CAD build for the part. Positions are in the model's coordinates, mm. Face numbers are marked on the shaded views. Round coordinates to 2 decimals unless told otherwise and drop trailing zeros. Loops run counter-clockwise (first coordinate to the right, second up) from the corner with the lowest first, then second, coordinate; pieces in that order, holes last. Notation, with made-up numbers: M 42.5,38 L 86.5,38 A37 ccw 86.5,75 Z; hole C -31.5,39.5 d8. An arc over 180 degrees is marked long. Use a Markdown table: item, result. Add a question column.
(1) Wall check: L1, parallel to Y at x = 33.25, z = 2.2; L2, parallel to Y at x = 23.5, z = 2.15; L3, parallel to X at y = -0.5, z = 2.8. Give the ranges that are in metal, low to high.
(2) Two-plate mould, pull along Y, no slides. Class the marked faces 1 and 2: released by +Y, released by -Y, zero draft, split by the parting line, or undercut.
(3) Band-saw the part on B-B, the plane x = 33.05. Write the cut outline in (y, z), and give its area (3 significant figures).
(4) Band-saw the part on D-D, the plane x = 12. Write the cut outline in (y, z), and give its area (3 significant figures).
(5) Band-saw the part on C-C, the plane z = 2.3. Give the number of separate pieces and of enclosed holes in the cut face, and give its area (3 significant figures).
(6) Band-saw the part on A-A, the plane y = -6. Write the cut outline in (x, z), and give its area (3 significant figures).
(7) Flat gauge pins, fed straight in: P1, Ø1.5, axis at y = -6, z = 1.5, coming from the -X side; P2, Ø1.5, axis at x = 39.5, z = 1.5, coming from the -Y side; P3, Ø1.5, axis at y = -5, z = 2, coming from the +X side. Where does each tip first touch, or does it go through?
from build123d import *

# Parameters (mm, degrees)
ESBO_O1_R                = 1.5
ESBO_O1_W                = 11
ESBO_O1_H                = 5.2
RESSALTO_EXTRUS_O1_DEPTH = 3
FILETE1_R                = 1.5
FILETE2_R                = 1.5


with BuildPart() as part:
    # Esboço1 → Ressalto-extrusão1 (new body)
    with BuildSketch(Plane.XY):
        with BuildLine():
            Line((0, 10.916708968), (0, 0))
            Line((0, 0), (3.1, 0))
            Line((3.1, 0), (3.1, -9))
            Line((3.1, -9), (11.2, -9))
            Line((11.2, -9), (11.2, 0))
            Line((11.2, 0), (29.2, 0))
            Line((29.2, 0), (29.2, -9))
            Line((29.2, -9), (37.3, -9))
            Line((37.3, -9), (37.3, 0))
            Line((37.3, 0), (40.4, 0))
            Line((40.4, 0), (40.4, 10.916708968))
            ThreePointArc((40.4, 10.916708968), (25, 14.2), (40.4, 17.483291032))
            Line((40.4, 17.483291032), (40.4, 28.4))
            Line((40.4, 28.4), (0, 28.4))
            Line((0, 28.4), (0, 17.483291032))
            ThreePointArc((0, 17.483291032), (9.028541033, 22.073055315), (15.4, 14.2))
            ThreePointArc((15.4, 14.2), (9.028541033, 6.326944685), (0, 10.916708968))
        make_face()
        with Locations((7.15, -6)):
            Circle(ESBO_O1_R, mode=Mode.SUBTRACT)
        with Locations((20.2, 6.6)):
            Rectangle(ESBO_O1_W, ESBO_O1_H, mode=Mode.SUBTRACT)
        with Locations((33.25, -6)):
            Circle(ESBO_O1_R, mode=Mode.SUBTRACT)
        with Locations((20.2, 21.8)):
            Rectangle(ESBO_O1_W, ESBO_O1_H, mode=Mode.SUBTRACT)
    extrude(amount=RESSALTO_EXTRUS_O1_DEPTH)

    # Filete1
    filete1_edges = [part.edges().sort_by_distance(p)[0] for p in [
        (14.7, 24.4, 1.5),
        (14.7, 19.2, 1.5),
        (25.7, 19.2, 1.5),
        (25.7, 24.4, 1.5),
    ]]
    fillet(filete1_edges, radius=FILETE1_R)

    # Filete2
    filete2_edges = [part.edges().sort_by_distance(p)[0] for p in [
        (25.7, 9.2, 1.5),
        (14.7, 9.2, 1.5),
        (14.7, 4, 1.5),
        (25.7, 4, 1.5),
    ]]
    fillet(filete2_edges, radius=FILETE2_R)


solid = part.part
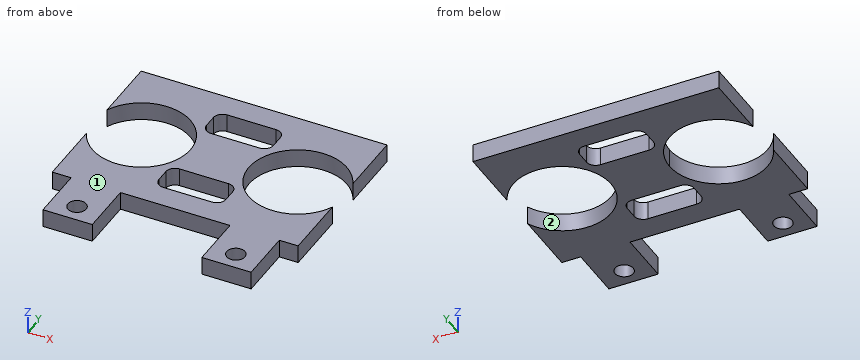
Return value:
| question | item | result |
|---|---|---|
| 1 | L1 | -9 to -7.5, -4.5 to 6.15, 22.25 to 28.4 |
| 1 | L2 | 0 to 4, 9.2 to 19.2, 24.4 to 28.4 |
| 1 | L3 | 3.1 to 11.2, 29.2 to 37.3 |
| 2 | face 1 | zero draft |
| 2 | face 2 | undercut |
| 3 | outline | M -9,0 L -7.49,0 L -7.49,3 L -9,3 Z; M -4.51,0 L 6.15,0 L 6.15,3 L -4.51,3 Z; M 22.25,0 L 28.4,0 L 28.4,3 L 22.25,3 Z |
| 3 | area | 55.0 mm^2 |
| 4 | outline | M 0,0 L 7.63,0 L 7.63,3 L 0,3 Z; M 20.77,0 L 28.4,0 L 28.4,3 L 20.77,3 Z |
| 4 | area | 45.8 mm^2 |
| 5 | separate pieces | 1 |
| 5 | enclosed holes | 4 |
| 5 | area | 768 mm^2 |
| 6 | outline | M 3.1,0 L 5.65,0 L 5.65,3 L 3.1,3 Z; M 8.65,0 L 11.2,0 L 11.2,3 L 8.65,3 Z; M 29.2,0 L 31.75,0 L 31.75,3 L 29.2,3 Z; M 34.75,0 L 37.3,0 L 37.3,3 L 34.75,3 Z |
| 6 | area | 30.6 mm^2 |
| 7 | P1 | x = 3.1 |
| 7 | P2 | y = 0 |
| 7 | P3 | x = 37.3 |
